Here's how the part is built. I have some questions about the finished solid (model axes, mm). Face numbers are marked on the shaded views. Round coordinates to 2 decimals unless told otherwise and drop trailing zeros. Order: outer loops, then holes, each group sorted by start corner. A loop starts at its lowest first (then second) coordinate and runs counter-clockwise, first axis right, second up. Notation, with made-up numbers: (1.25, -7) -> (44.25, -7) arc R29 cw to (44.25, 32) -> close; hole circle Ø11 at (11, -34.75). An arc over 180 degrees is marked (long way). One line per item, written item: value.
```python
from build123d import *

# Parameters (mm, degrees)
SKETCH_W        = 25
SKETCH_H        = 60
PAD_DEPTH       = 5
POCKET_DEPTH    = 2.5
SKETCH002_R     = 1.8
POCKET001_DEPTH = 1.8


with BuildPart() as part:
    # Sketch → Pad (new body)
    with BuildSketch(Plane.XY):
        with Locations((17.5, 30)):
            Rectangle(SKETCH_W, SKETCH_H)
    extrude(amount=PAD_DEPTH)

    # Sketch001 → Pocket (cut)
    with BuildSketch(Plane.XY.offset(5)):
        with BuildLine():
            ThreePointArc((27.5, 45.004765), (15, 57.504765), (2.5, 45.004764))
            Line((2.5, 45.004764), (2.5, 15.004765))
            ThreePointArc((2.5, 15.004765), (15, 2.504765), (27.5, 15.004765))
            Line((27.5, 15.004765), (27.5, 45.004765))
        make_face()
        with BuildLine():
            ThreePointArc((22.5, 45.004765), (15, 52.504765), (7.5, 45.004765))
            Line((7.5, 45.004765), (7.5, 15.004765))
            ThreePointArc((7.5, 15.004765), (15, 7.504765), (22.5, 15.004765))
            Line((22.5, 45.004765), (22.5, 15.004765))
        make_face(mode=Mode.SUBTRACT)
    extrude(amount=-POCKET_DEPTH, mode=Mode.SUBTRACT)

    # Sketch002 → Pocket001 (cut)
    with BuildSketch(Plane.XY.offset(5)):
        with Locations((15, 45)):
            Circle(SKETCH002_R)
        with Locations((15, 15)):
            Circle(SKETCH002_R)
    extrude(amount=-POCKET001_DEPTH, mode=Mode.SUBTRACT)


solid = part.part
```
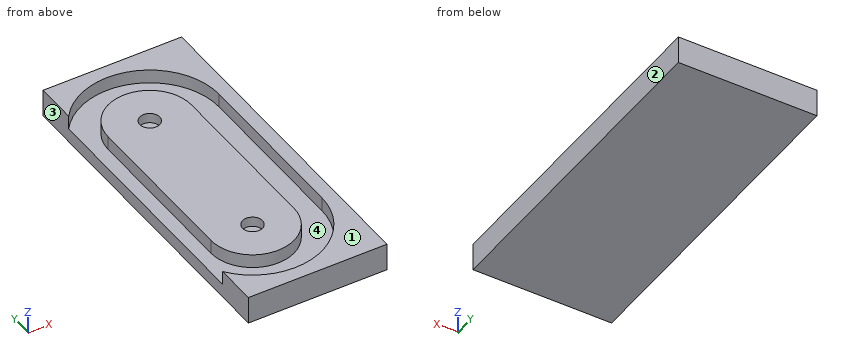
Q1. If we mould it in two halves opening along X, with no side actions, what happens to the marked faces 1, 2, 3 and 4? For each: pulls with the +X half, pulls with the -X half, needs draft (parallel to the pull), parting line crosses it, or undercut.
Answers:
face 1: needs draft
face 2: pulls with the +X half
face 3: pulls with the -X half
face 4: undercut
Q2. I need wall thicknesses on line 1 along Y through (x, z) = (15, 3.95); line 2 along Y through (x, z) = (11.25, 4.25); line 3 along Y through (x, z) = (13.5, 3.35). Which ranges of each line are inside material? Lowest first, please.
Answers:
line 1: 0 to 2.5, 7.5 to 13.2, 16.8 to 43.2, 46.8 to 52.5, 57.5 to 60
line 2: 0 to 3.08, 8.51 to 51.5, 56.93 to 60
line 3: 0 to 2.6, 7.66 to 14.01, 15.99 to 44.01, 45.99 to 52.35, 57.41 to 60
Q3. For P1, Ø2, axis at y = 25.5, z = 4, coming from the -X side; P2, Ø1.8, axis at x = 14.5, y = 14.5, coming from the +Z side, each with a flat end and sliding along its axis, tell me the tip position at first contact or that it passes through.
Answers:
P1: x = 7.5
P2: z = 3.2
Q4. I want a section at B-B on y = 22.5. Write out the boundary of the cut face in (x, z), then the cut area to 3 significant figures.
Answers:
outline: (5, 0) -> (30, 0) -> (30, 5) -> (27.5, 5) -> (27.5, 2.5) -> (22.5, 2.5) -> (22.5, 5) -> (7.5, 5) -> (7.5, 2.5) -> (5, 2.5) -> close
area: 106 mm2
Q5. I want a section at A-A on z = 4. Write out the boundary of the cut face in (x, y).
Answers:
outline: (5, 0) -> (30, 0) -> (30, 60) -> (5, 60) -> (5, 52.5) arc R12.5 cw to (27.5, 45) -> (27.5, 15) arc R12.5 cw to (5, 7.5) -> close; (7.5, 15) arc R7.5 ccw to (22.5, 15) -> (22.5, 45) arc R7.5 ccw to (7.5, 45) -> close; hole circle Ø3.6 at (15, 15); hole circle Ø3.6 at (15, 45)
Q6. I want a section at C-C on x = 15. Write out the boundary of the cut face in (y, z).
Answers:
outline: (0, 0) -> (60, 0) -> (60, 5) -> (57.5, 5) -> (57.5, 2.5) -> (52.5, 2.5) -> (52.5, 5) -> (46.8, 5) -> (46.8, 3.2) -> (43.2, 3.2) -> (43.2, 5) -> (16.8, 5) -> (16.8, 3.2) -> (13.2, 3.2) -> (13.2, 5) -> (7.5, 5) -> (7.5, 2.5) -> (2.5, 2.5) -> (2.5, 5) -> (0, 5) -> close
Q7. I want a section at D-D on y = 16. Write out the boundary of the cut face in (x, z), then the cut area to 3 significant figures.
Answers:
outline: (5, 0) -> (30, 0) -> (30, 5) -> (27.5, 5) -> (27.5, 2.5) -> (22.5, 2.5) -> (22.5, 5) -> (16.5, 5) -> (16.5, 3.2) -> (13.5, 3.2) -> (13.5, 5) -> (7.5, 5) -> (7.5, 2.5) -> (5, 2.5) -> close
area: 101 mm2
